Read the model definition and answer for the solid it produces. Units are mm, in the model's axes. Coordinates: 2 decimals unless noted, no trailing zeros. Loops run counter-clockwise (first coordinate to the right, second up) from the corner with the lowest first, then second, coordinate; pieces in that order, holes last. Notation, with made-up numbers: (85, 80) -> (105, 80) arc R16 cw to (105, 95) -> close; hole circle Ø1 at (44, 4.25). An arc over 180 degrees is marked (long way). Answer in a Markdown table with one row per item.
```python
from build123d import *

# Parameters (mm, degrees)
SKETCH1_W           = 60
SKETCH1_H           = 50
BOSS_EXTRUDE1_DEPTH = 4.76
SKETCH2_R           = 1.65
SKETCH2_R_2         = 3.25
CUT_EXTRUDE1_DEPTH  = 5.76
FILLET1_R           = 10
FILLET2_R           = 5


with BuildPart() as part:
    # Sketch1 → Boss-Extrude1 (new body)
    with BuildSketch(Plane.XY):
        with Locations((30, 25)):
            Rectangle(SKETCH1_W, SKETCH1_H)
    extrude(amount=BOSS_EXTRUDE1_DEPTH)

    # Sketch2 → Cut-Extrude1 (cut, through all)
    with BuildSketch(Plane.XY.offset(4.76)):
        with Locations((10, 12.5)):
            Circle(SKETCH2_R)
        with Locations((50, 12.5)):
            Circle(SKETCH2_R)
        with Locations((30, 40)):
            Circle(SKETCH2_R_2)
    extrude(amount=-CUT_EXTRUDE1_DEPTH, mode=Mode.SUBTRACT)

    # Fillet1
    fillet1_edges = [part.edges().sort_by_distance(p)[0] for p in [
        (0, 50, 2.38),
        (60, 50, 2.38),
    ]]
    fillet(fillet1_edges, radius=FILLET1_R)

    # Fillet2
    fillet2_edges = [part.edges().sort_by_distance(p)[0] for p in [
        (60, 0, 2.38),
        (0, 0, 2.38),
    ]]
    fillet(fillet2_edges, radius=FILLET2_R)


solid = part.part
```
1. The mould has two halves that part along X. Classify faces 1 (the flat face through (60, 22, 2)), 2 (the flat face through (30, 25, 4.76)), 3 (the cylindrical face through (31.5, 37.117, 2.413)): pulls with the +X half, pulls with the -X half, needs draft (parallel to the pull), parting line crosses it, or undercut.
A:
| item | result |
|---|---|
| face 1 | pulls with the +X half |
| face 2 | needs draft |
| face 3 | undercut |
2. A cutting plane is placed at D-D on y = 45.5. Give the vertices of the cut face in (x, z).
A:
| item | result |
|---|---|
| outline | (1.65, 0) -> (58.35, 0) -> (58.35, 4.76) -> (1.65, 4.76) -> close |
3. A cutting plane is placed at A-A on y = 12.5. Give the vertices of the cut face in (x, z).
A:
| item | result |
|---|---|
| outline | (0, 0) -> (8.35, 0) -> (8.35, 4.76) -> (0, 4.76) -> close; (11.65, 0) -> (48.35, 0) -> (48.35, 4.76) -> (11.65, 4.76) -> close; (51.65, 0) -> (60, 0) -> (60, 4.76) -> (51.65, 4.76) -> close |
4. Find the intervals of material crossed by probe 1 along Y at (x, z) = (30, 3.4); probe 2 along Y at (x, z) = (10, 3); probe 3 along X at (y, z) = (37, 4.5), in increasing order.
A:
| item | result |
|---|---|
| probe 1 | y = 0 to 36.75, 43.25 to 50 |
| probe 2 | y = 0 to 10.85, 14.15 to 50 |
| probe 3 | x = 0 to 28.75, 31.25 to 60 |
5. A cutting plane is placed at B-B on z = 2.55. Give the vertices of the cut face in (x, y), and give its area (3 significant figures).
A:
| item | result |
|---|---|
| outline | (0, 5) arc R5 ccw to (5, 0) -> (55, 0) arc R5 ccw to (60, 5) -> (60, 40) arc R10 ccw to (50, 50) -> (10, 50) arc R10 ccw to (0, 40) -> close; hole circle Ø3.3 at (10, 12.5); hole circle Ø6.5 at (30, 40); hole circle Ø3.3 at (50, 12.5) |
| area | 2,900 mm2 |
6. A cutting plane is placed at C-C on x = 29.5. Give the vertices of the cut face in (y, z).
A:
| item | result |
|---|---|
| outline | (0, 0) -> (36.79, 0) -> (36.79, 4.76) -> (0, 4.76) -> close; (43.21, 0) -> (50, 0) -> (50, 4.76) -> (43.21, 4.76) -> close |
